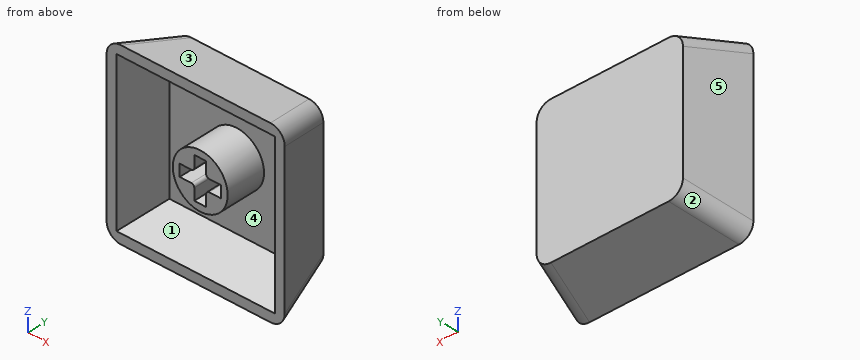
Autodesk Inventor part; units mm, degrees
ref_plane "Work Plane1" through (-9, 33.5885, 16.5511) normal (1, 0, 0) x (0, 0, -1)
ref_plane "YZ Plane" through (0, 0, 0) normal (1, 0, 0) x (0, 1, 0)
ref_plane "XZ Plane" through (0, 0, 0) normal (0, 1, 0) x (-1, 0, 0)
sketch "Sketch1" plane through (0, 0, 0) normal (0, 1, 0) x (-1, 0, 0)
  line L0 (0, 0) -> (18, 0)
  line L1 (18, 0) -> (18, 18)
  line L2 (18, 18) -> (0, 18)
  line L3 (0, 18) -> (0, 0)
  dimension "d0" = 18
  dimension "d1" = 18
extrude "Extrusion1" add sketch "Sketch1" along normal blind 8 draft -15
fillet "Fillet1" radius 1.5 8 edges at (-1.0718, 4, 16.9282) (-9, 8, 15.8564) (-2.1436, 8, 9) (-9, 8, 2.1436) (-1.0718, 4, 1.0718) (-16.9282, 4, 1.0718) (-16.9282, 4, 16.9282) (-15.8564, 8, 9)
ref_plane "Work Plane1" through (-9, 33.5885, 16.5511) normal (1, 0, 0) x (0, 0, -1)
sketch "Sketch2" plane through (-9, 33.5885, 16.5511) normal (1, 0, 0) x (0, 0, -1)
  line L0 (13.2565, -25.5885) -> (1.8457, -25.5885)
  arc A0 (14.7054, -26.7002) -> (13.2565, -25.5885) centre (13.2565, -27.0885) ccw
  arc A1 (1.8457, -25.5885) -> (13.2565, -25.5885) centre (7.5511, -8.5166) ccw
  point P0 (16.5511, -33.5885)
  point P1 (13.2565, -25.5885)
  dimension "d5" = 18
extrude "Extrusion2" cut sketch "Sketch2" along normal through all both and the other way through all
sketch "Sketch3" plane through (0, 0, 0) normal (0, -1, 0) x (1, 0, 0)
  line L0 (-16.5511, 18) -> (-1.4489, 18) construction
  line L1 (-9, 18) -> (-9, 0) construction
  line L2 (-1.4489, 0) -> (-16.5511, 0) construction
  line L3 (-18, 1.4489) -> (-18, 16.5511) construction
  line L4 (-18, 9) -> (0, 9) construction
  line L5 (-1, 1) -> (-17, 1)
  line L6 (-17, 1) -> (-17, 17)
  line L7 (-17, 17) -> (-1, 17)
  line L8 (-1, 17) -> (-1, 1)
  line L9 (-1, 1) -> (-17, 17) construction
  line L10 (-17, 1) -> (-1, 17) construction
  point P0 (0, 0)
  point P1 (-9, 9)
  point P2 (-9, 9)
  dimension "d8" = 16
  dimension "d9" = 16
extrude "Extrusion3" cut sketch "Sketch3" against normal blind 4.5 draft -15
sketch "Sketch4" plane through (0, 4.5, 0) normal (0, -1, 0) x (1, 0, 0)
  line L0 (-15.7942, 15.7942) -> (-15.7942, 2.2058) construction
  line L1 (-15.7942, 9) -> (-2.2058, 9) construction
  line L2 (-2.2058, 2.2058) -> (-2.2058, 15.7942) construction
  line L3 (-2.2058, 15.7942) -> (-15.7942, 15.7942) construction
  line L4 (-9, 15.7942) -> (-9, 2.2058) construction
  line L5 (-15.7942, 2.2058) -> (-2.2058, 2.2058) construction
  circle A0 centre (-9, 9) radius 2.775
  point P0 (0, 0)
  dimension "d12" = 5.55
extrude "Extrusion4" add sketch "Sketch4" along normal blind 4
sketch "Sketch5" plane through (-9, 0.5, 9) normal (0, -1, 0) x (1, 0, 0)
  line L0 (0.6, 2.075) -> (-0.6, 2.075)
  line L1 (-0.6, -2.075) -> (0.6, -2.075)
  line L2 (-0.6, 2.075) -> (0.6, -2.075) construction
  line L3 (-2.075, 0.6) -> (-2.075, -0.6)
  line L4 (2.075, -0.6) -> (2.075, 0.6)
  line L5 (2.075, 0.6) -> (-2.075, -0.6) construction
  line L6 (-2.075, 0.6) -> (2.075, -0.6) construction
  line L7 (-6.7942, 6.7942) -> (-6.7942, -6.7942) construction
  line L8 (-6.7942, 0) -> (6.7942, 0) construction
  line L9 (6.7942, -6.7942) -> (6.7942, 6.7942) construction
  line L10 (-6.7942, -6.7942) -> (6.7942, -6.7942) construction
  line L11 (0, -6.7942) -> (0, 6.7942) construction
  arc A0 (0.9, -0.6) -> (0.6, -0.9) centre (0.9, -0.9) ccw
  arc A1 (-0.6, -0.9) -> (-0.9, -0.6) centre (-0.9, -0.9) ccw
  arc A2 (0.6, 0.9) -> (0.9, 0.6) centre (0.9, 0.9) ccw
  arc A3 (-0.9, 0.6) -> (-0.6, 0.9) centre (-0.9, 0.9) ccw
  line L12 (-0.6, 2.075) -> (-0.6, 0.9)
  line L13 (-0.6, -0.9) -> (-0.6, -2.075)
  line L14 (-2.075, -0.6) -> (-0.9, -0.6)
  line L15 (-0.9, 0.6) -> (-2.075, 0.6)
  line L16 (0.6, 2.075) -> (0.1735, 0.6) construction
  line L17 (0, 0) -> (-0.6, -2.075) construction
  line L18 (2.075, 0.6) -> (0.9, 0.6)
  line L19 (0.9, -0.6) -> (2.075, -0.6)
  line L20 (0.6, -2.075) -> (0.6, -0.9)
  line L21 (0.6, 0.9) -> (0.6, 2.075)
  point P0 (9, -9)
  dimension "d15" = 1.2
  dimension "d16" = 4.15
  dimension "d17" = 4.15
  dimension "d18" = 1.2
  dimension "d19" = 0.3
extrude "Extrusion5" cut sketch "Sketch5" against normal blind 4
ref_plane "Work Plane3" through (0, 6, 0) normal (0, -1, 0) x (1, 0, 0)
split_face "Split1"
sketch "Sketch7" plane through (0, 6, 0) normal (0, -1, 0) x (1, 0, 0)
  line L0 (-25.6931, 27.6788) -> (12.1363, 27.6788)
  line L1 (12.1363, 27.6788) -> (12.1363, -37.3947)
  line L2 (12.1363, -37.3947) -> (-25.6931, -37.3947)
  line L3 (-25.6931, -37.3947) -> (-25.6931, 27.6788)
  point P0 (0, 0)
extrude "Extrusion7" cut sketch "Sketch7" against normal blind 10
properties part number "bottom"
The model under review builds one solid part; all positions refer to its coordinate system, in mm. Face numbers are marked on the shaded views. A direction names the side the tool comes from. Coordinates: 2 decimals unless noted, no trailing zeros. Loops run counter-clockwise (first coordinate to the right, second up) from the corner with the lowest first, then second, coordinate; pieces in that order, holes last. Notation, with made-up numbers: M 89,-15.75 L 117,-15.75 A22 cw 117,22.25 Z; hole C 68.25,-9 d6. An arc over 180 degrees is marked long. Put each result on its own line as item: value. Start each with the question number.
Q1. For the marked faces 4 and 5, list the 3-axis set-ups (+Z, -Z, +X, -X, +Y, -Y) from which the entire face can be reached by the end or side of a thin tool; tool diameter is ignored.
Q2. Add section C-C (z = 13.25). Write out the cut boundary in (x, y), and give its area (3 significant figures).
Q3. Add section B-B (y = 2.25). Count the separate pieces of the cut face and the enclosed holes in it, and give its area (3 significant figures).
Q4. The part is to be moulded in two halves that separate along Z. For the marked faces 1, 2 and 3, say which applies: +Z half, -Z half, draft (parallel to the pull), parting line (faces both ways), or undercut.
Q5. Clearance check with flat-ended pins moving along their axes: pin 1 (0.9 mm diameter, centred on y = 3, z = 7.5, fed in from -X); pin 2 (0.9 mm diameter, centred on x = -7.5, y = 2, fed in from +Z); pin 3 (4 mm diameter, centred on x = -11, z = 11.5, fed in from -Y). State where each tip first meets the part, or that it passes through.
Q6. Add section A-A (x = -9). Write out the cut boundary in (y, z) (3 decimals), and give its area (3 significant figures).
Q7. Wall thickness on line 1 (Z direction, x = -8, y = 2.25); line 2 (Z direction, x = -9.75, y = 4); line 3 (X direction, y = 3.25, z = 7.25): over which ranges is each line inside the solid? List them lowest first.
Q8. Add section D-D (x = -14). Write out the cut boundary in (y, z), and give its area (3 significant figures).
Answers:
1. face 4: -Y
1. face 5: +Z, -Z, -X, +Y
2. outline: M -18,0 L -17,0 L -15.79,4.5 L -2.21,4.5 L -1,0 L 0,0 L -1.61,6 L -16.39,6 Z
2. area: 31.8 mm^2
3. separate pieces: 2
3. enclosed holes: 2
3. area: 77.0 mm^2
4. face 1: undercut
4. face 2: -Z half
4. face 3: +Z half
5. pin 1: stops at x = -17.32
5. pin 2: stops at z = 17.58
5. pin 3: stops at y = 0.5
6. outline: M 0,0 L 6,1.608 L 6,16.392 L 0,18 L 0,17 L 4.5,15.794 L 4.5,11.775 L 0.5,11.775 L 0.5,11.075 L 4.5,11.075 L 4.5,6.925 L 0.5,6.925 L 0.5,6.225 L 4.5,6.225 L 4.5,2.206 L 0,1 Z
6. area: 37.4 mm^2
7. line 1: z = 0.6 to 1.6, 6.41 to 8.4, 9.6 to 11.59, 16.4 to 17.4
7. line 2: z = 1.07 to 2.07, 6.33 to 8.36, 9.64 to 11.67, 15.93 to 16.93
7. line 3: x = -17.13 to -16.13, -11.15 to -9.6, -8.4 to -6.85, -1.87 to -0.87
8. outline: M 0,0 L 6,1.61 L 6,16.39 L 0,18 L 0,17 L 4.5,15.79 L 4.5,2.21 L 0,1 Z
8. area: 31.8 mm^2
